from build123d import *

# Parameters (mm, degrees)
F0_R     = 12
F0_R_2   = 6
F1_DEPTH = 30
F2_W     = 30
F2_H     = 15
F3_DEPTH = 12.5
F4_R     = 2.5
F5_DEPTH = 12.5


with BuildPart() as f1:
    # F0 (on Front) → F1 (new body)
    with BuildSketch(Plane.XZ):
        Circle(F0_R)
        Circle(F0_R_2, mode=Mode.SUBTRACT)
    extrude(amount=F1_DEPTH)

    # F2 (on Right) → F3 (cut, symmetric)
    with BuildSketch(Plane.YZ):
        Rectangle(F2_W, F2_H)
    extrude(amount=F3_DEPTH, both=True, mode=Mode.SUBTRACT)

    # F4 (on Top) → F5 (cut, symmetric)
    with BuildSketch(Plane.XY):
        with Locations((0, -4.5)):
            Circle(F4_R)
    extrude(amount=F5_DEPTH, both=True, mode=Mode.SUBTRACT)


solid = f1.part
Could you check a few things on this model? Use its own coordinates, in mm. A direction names the side the tool comes from. Give positions to 0.01 mm unless a question says otherwise; leave off trailing zeros. Order: outer loops, then holes, each group sorted by start corner. A loop starts at its lowest first (then second) coordinate and runs counter-clockwise, first axis right, second up.
1. Suppose I cut it at B-B (x = 0). Write out the boundary of the cut face in (y, z).
Answers below:
outline: (-30, -12) - (-7, -12) - (-7, -7.5) - (-15, -7.5) - (-15, -6) - (-30, -6) - close; (-30, 6) - (-15, 6) - (-15, 7.5) - (-7, 7.5) - (-7, 12) - (-30, 12) - close; (-2, -12) - (0, -12) - (0, -7.5) - (-2, -7.5) - close; (-2, 7.5) - (0, 7.5) - (0, 12) - (-2, 12) - close
2. I need wall thicknesses on L1, parallel to Y at x = 0, z = 9.35; L2, parallel to X at y = -19.5, z = 0. Which ranges of each line are inside material? Lowest first, please.
Answers below:
L1: y = -30 to -7, -2 to 0
L2: x = -12 to -6, 6 to 12
3. Thinking about a two-plate mould opening in Z: for faces 1 (the cylindrical face through (-1.56, -18.12, 11.9)), 2 (the cylindrical face through (-6, -22, 0)), 3 (the cylindrical face through (-2.5, -4.4, 9.8)), which applies, +Z half, -Z half, draft (parallel to the pull), parting line (faces both ways), or undercut?
Answers below:
face 1: parting line
face 2: undercut
face 3: draft
4. Suppose I cut it at A-A (z = 0). Write out the boundary of the cut face in (x, y), plus the area to 3 significant figures.
Answers below:
outline: (-12, -30) - (-6, -30) - (-6, -15) - (-12, -15) - close; (6, -30) - (12, -30) - (12, -15) - (6, -15) - close
area: 180 mm2
5. For pin 1 (12 mm diameter, centred on x = 4.5, y = -7, fed in from +Z); pin 2 (2 mm diameter, centred on x = -2, y = -3.5, fed in from -Z); pin 3 (11 mm diameter, centred on x = 0, z = 0, fed in from -Y); pin 4 (7.5 mm diameter, centred on x = -3, z = 0, fed in from +Y), each with a flat end and sliding along its axis, tell me the tip position at first contact or that it passes through.
Answers below:
pin 1: stops at z = 12
pin 2: stops at z = -11.89
pin 3: passes through
pin 4: stops at y = -15
6. Which directions (+Z, -Z, +X, -X, +Y, -Y) give clear straight access to the entire face, cutting with the end or side of a thin tool? Please do faces 4 (the flat face through (0, -8, 7.5)), 5 (the cylindrical face through (0, -2, -10)).
Answers below:
face 4: +X, -X, +Y
face 5: +Z, -Z
7. Suppose I cut it at D-D (y = -4.5). Write out the boundary of the cut face in (x, z).
Answers below:
outline: (-9.37, -7.5) arc R12 ccw to (-2.5, -11.74) - (-2.5, -7.5) - close; (-9.37, 7.5) - (-2.5, 7.5) - (-2.5, 11.74) arc R12 ccw to start; (2.5, -11.74) arc R12 ccw to (9.37, -7.5) - (2.5, -7.5) - close; (2.5, 7.5) - (9.37, 7.5) arc R12 ccw to (2.5, 11.74) - close
8. Suppose I cut it at C-C (x = 5.25). Write out the boundary of the cut face in (y, z).
Answers below:
outline: (-30, -10.79) - (0, -10.79) - (0, -7.5) - (-15, -7.5) - (-15, -2.9) - (-30, -2.9) - close; (-30, 2.9) - (-15, 2.9) - (-15, 7.5) - (0, 7.5) - (0, 10.79) - (-30, 10.79) - close
